```python
from build123d import *

# Parameters (mm, degrees)
SKETCH1_R           = 15.875
BOSS_EXTRUDE1_DEPTH = 52.5
CHAMFER1_SIZE       = 2
SKETCH2_R           = 15.875
SKETCH2_R_2         = 14.875
CUT_EXTRUDE1_DEPTH  = 2


with BuildPart() as part:
    # Sketch1 → Boss-Extrude1 (new body, symmetric)
    with BuildSketch(Plane(origin=(0, 0, 0), x_dir=(0, 0, -1), z_dir=(1, 0, 0))):
        Circle(SKETCH1_R)
    extrude(amount=BOSS_EXTRUDE1_DEPTH, both=True)

    # Chamfer1
    chamfer1_edges = [part.edges().sort_by_distance(p)[0] for p in [
        (-52.5, 0, 15.875),
        (52.5, 0, 15.875),
    ]]
    chamfer(chamfer1_edges, length=CHAMFER1_SIZE)

    # Sketch2 → Cut-Extrude1 (cut)
    with BuildSketch(Plane.ZY.offset(47.5)):
        Circle(SKETCH2_R)
        Circle(SKETCH2_R_2, mode=Mode.SUBTRACT)
    cut_extrude1 = extrude(amount=CUT_EXTRUDE1_DEPTH, mode=Mode.SUBTRACT)

    # Mirror1: Cut-Extrude1 across plane
    add(cut_extrude1.mirror(Plane(origin=(0, 0, 0), x_dir=(0, 0, 1), z_dir=(1, 0, 0))), mode=Mode.SUBTRACT)


solid = part.part
```
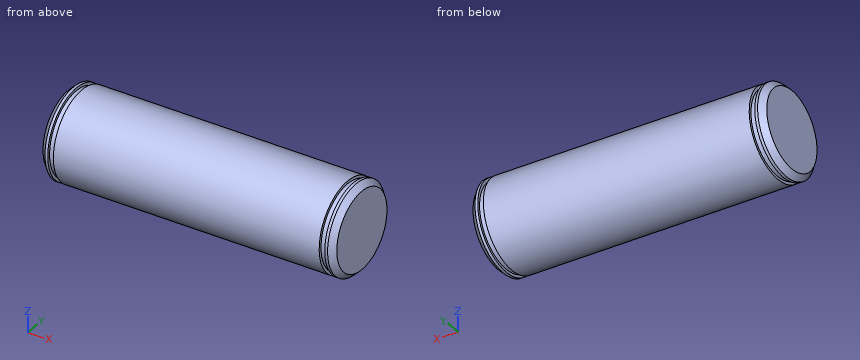
Here's how the part is built. I have some questions about the finished solid (model axes, mm). Round coordinates to 2 decimals unless told otherwise and drop trailing zeros. Loops run counter-clockwise (first coordinate to the right, second up) from the corner with the lowest first, then second, coordinate; pieces in that order, holes last.
1. Will these pins go through, and if not, where does the flat tip stop? pin 1 (4 mm diameter, centred on x = 11.5, y = 2, fed in from -Z) (3 decimals); pin 2 (3 mm diameter, centred on x = -42, y = 8, fed in from +Z); pin 3 (3 mm diameter, centred on x = -39.5, z = -8.5, fed in from +Y); pin 4 (1 mm diameter, centred on x = 38, y = 8.5, fed in from +Z).
Answers:
pin 1: stops at z = -15.875
pin 2: stops at z = 14.48
pin 3: stops at y = 14.25
pin 4: stops at z = 13.71
2. Suppose I cut it at A-A, the plane x = -24. Please give me the cut outline in (y, z) (3 decimals).
Answers:
outline: circle Ø31.75 at (0, 0)
3. If I drill on probe 1 along Y at (x, z) = (24.5, -9.5); probe 2 along X at (y, z) = (-2, 14); probe 3 along Y at (x, z) = (-12, -9), over which ranges is the centre line in solid material (lowest first)?
Answers:
probe 1: y = -12.72 to 12.72
probe 2: x = -52.23 to 52.23
probe 3: y = -13.08 to 13.08
